```python
from build123d import *

# Parameters (mm, degrees)
BOSS_EXTRUDE1_DEPTH = 50
CUT_EXTRUDE1_REACH  = 129.279
SKETCH3_R           = 5.716504826
CUT_EXTRUDE2_REACH  = 124.474
SKETCH5_R           = 2.5


with BuildPart() as part:
    # Sketch2 → Boss-Extrude1 (new body)
    with BuildSketch(Plane(origin=(0, 0, 0), x_dir=(1, 0, 0), z_dir=(0, 1, 0))):
        Polygon((0, 0), (110, 0), (110, 50), (100, 50), (100, 10), (0, 10), align=None)
    extrude(amount=BOSS_EXTRUDE1_DEPTH)

    # Sketch3 → Cut-Extrude1 (cut, up to next)
    with BuildSketch(Plane(origin=(0, 0, -10), x_dir=(-1, 0, 0), z_dir=(0, 0, -1)), mode=Mode.PRIVATE) as cut_extrude1_sk1:
        with Locations((-50, 25)):
            Circle(SKETCH3_R)
    cut_extrude1_tool1 = extrude(cut_extrude1_sk1.sketch, amount=-CUT_EXTRUDE1_REACH, mode=Mode.PRIVATE) & part.part
    add(cut_extrude1_tool1.solids().sort_by_distance((50, 25, -10))[0], mode=Mode.SUBTRACT)

    # Sketch5 → Cut-Extrude2 (cut, up to next)
    with BuildSketch(Plane.ZY.offset(-100), mode=Mode.PRIVATE) as cut_extrude2_sk1:
        with Locations((-40, 12.5)):
            Circle(SKETCH5_R)
    cut_extrude2_tool1 = extrude(cut_extrude2_sk1.sketch, amount=-CUT_EXTRUDE2_REACH, mode=Mode.PRIVATE) & part.part
    # Sketch5 → Cut-Extrude2 (cut, up to next)
    with BuildSketch(Plane.ZY.offset(-100), mode=Mode.PRIVATE) as cut_extrude2_sk2:
        with Locations((-20, 12.5)):
            Circle(SKETCH5_R)
    cut_extrude2_tool2 = extrude(cut_extrude2_sk2.sketch, amount=-CUT_EXTRUDE2_REACH, mode=Mode.PRIVATE) & part.part
    # Sketch5 → Cut-Extrude2 (cut, up to next)
    with BuildSketch(Plane.ZY.offset(-100), mode=Mode.PRIVATE) as cut_extrude2_sk3:
        with Locations((-40, 37.5)):
            Circle(SKETCH5_R)
    cut_extrude2_tool3 = extrude(cut_extrude2_sk3.sketch, amount=-CUT_EXTRUDE2_REACH, mode=Mode.PRIVATE) & part.part
    # Sketch5 → Cut-Extrude2 (cut, up to next)
    with BuildSketch(Plane.ZY.offset(-100), mode=Mode.PRIVATE) as cut_extrude2_sk4:
        with Locations((-20, 37.5)):
            Circle(SKETCH5_R)
    cut_extrude2_tool4 = extrude(cut_extrude2_sk4.sketch, amount=-CUT_EXTRUDE2_REACH, mode=Mode.PRIVATE) & part.part
    add(cut_extrude2_tool1.solids().sort_by_distance((100, 12.5, -40))[0], mode=Mode.SUBTRACT)
    add(cut_extrude2_tool2.solids().sort_by_distance((100, 12.5, -20))[0], mode=Mode.SUBTRACT)
    add(cut_extrude2_tool3.solids().sort_by_distance((100, 37.5, -40))[0], mode=Mode.SUBTRACT)
    add(cut_extrude2_tool4.solids().sort_by_distance((100, 37.5, -20))[0], mode=Mode.SUBTRACT)


solid = part.part
```
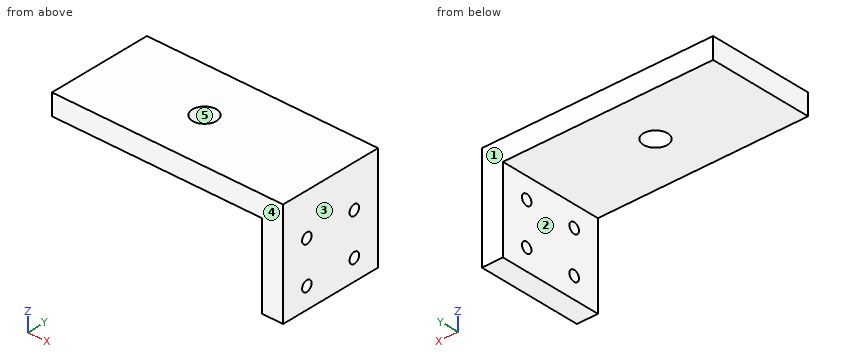
Read the model definition and answer for the solid it produces. Units are mm, in the model's axes. Face numbers are marked on the shaded views. A direction names the side the tool comes from. Coordinates: 2 decimals unless noted, no trailing zeros. Loops run counter-clockwise (first coordinate to the right, second up) from the corner with the lowest first, then second, coordinate; pieces in that order, holes last.
(1) The mould has two halves that part along Y. Classify the marked faces 3, 4 and 5: released by +Y, released by -Y, zero draft, split by the parting line, or undercut.
Solution:
face 3: zero draft
face 4: released by -Y
face 5: undercut
(2) The part is cut by section A-A (y = 37.5). Determine the outline of the cut face in (x, z), and give its area (3 significant figures).
Solution:
outline: (0, -10) - (100, -10) - (100, -17.5) - (110, -17.5) - (110, 0) - (0, 0) - close; (100, -50) - (110, -50) - (110, -42.5) - (100, -42.5) - close; (100, -37.5) - (110, -37.5) - (110, -22.5) - (100, -22.5) - close
area: 1,400 mm2
(3) A tool of negligible diameter and unlimited length cuts with its end or side. For the marked faces 1 and 2, from which of +Z, -Z, +X, -X, +Y, -Y can it reach the whole face along a straight path? Write none if from no direction.
Solution:
face 1: +Z, -Z, +X, -X, +Y
face 2: -Z, -X, +Y, -Y
(4) Consider line 1 along Y through (x, z) = (107, -40); line 2 along Z through (x, y) = (105, 12); line 3 along X through (y, z) = (4, -20.5). Determine where each line is inside the solid, lowest interval first.
Solution:
line 1: y = 0 to 10, 15 to 35, 40 to 50
line 2: z = -50 to -42.45, -37.55 to -22.45, -17.55 to 0
line 3: x = 100 to 110
(5) Flat-ended cylindrical pins translate along their axes: pin 1 Ø8 at (y, z) = (39.5, -15) entering from -X; pin 2 Ø1.5 at (x, y) = (39, 12.5) entering from -Z; pin 3 Ø7 at (x, y) = (50, 25) entering from +Z. Find the tip coordinate at first contact, or state that the pin passes through.
Solution:
pin 1: stops at x = 100
pin 2: stops at z = -10
pin 3: passes through
(6) The part is cut by section B-B (z = -20). Determine the outline of the cut face in (x, y).
Solution:
outline: (100, 0) - (110, 0) - (110, 10) - (100, 10) - close; (100, 15) - (110, 15) - (110, 35) - (100, 35) - close; (100, 40) - (110, 40) - (110, 50) - (100, 50) - close
(7) The part is cut by section C-C (y = 25). Determine the outline of the cut face in (x, z), and give its area (3 significant figures).
Solution:
outline: (0, -10) - (44.28, -10) - (44.28, 0) - (0, 0) - close; (55.72, -10) - (100, -10) - (100, -50) - (110, -50) - (110, 0) - (55.72, 0) - close
area: 1,390 mm2
(8) The part is cut by section D-D (z = -8.5). Determine the outline of the cut face in (x, y), and give its area (3 significant figures).
Solution:
outline: (0, 0) - (110, 0) - (110, 50) - (0, 50) - close; hole circle Ø11.43 at (50, 25)
area: 5,400 mm2
